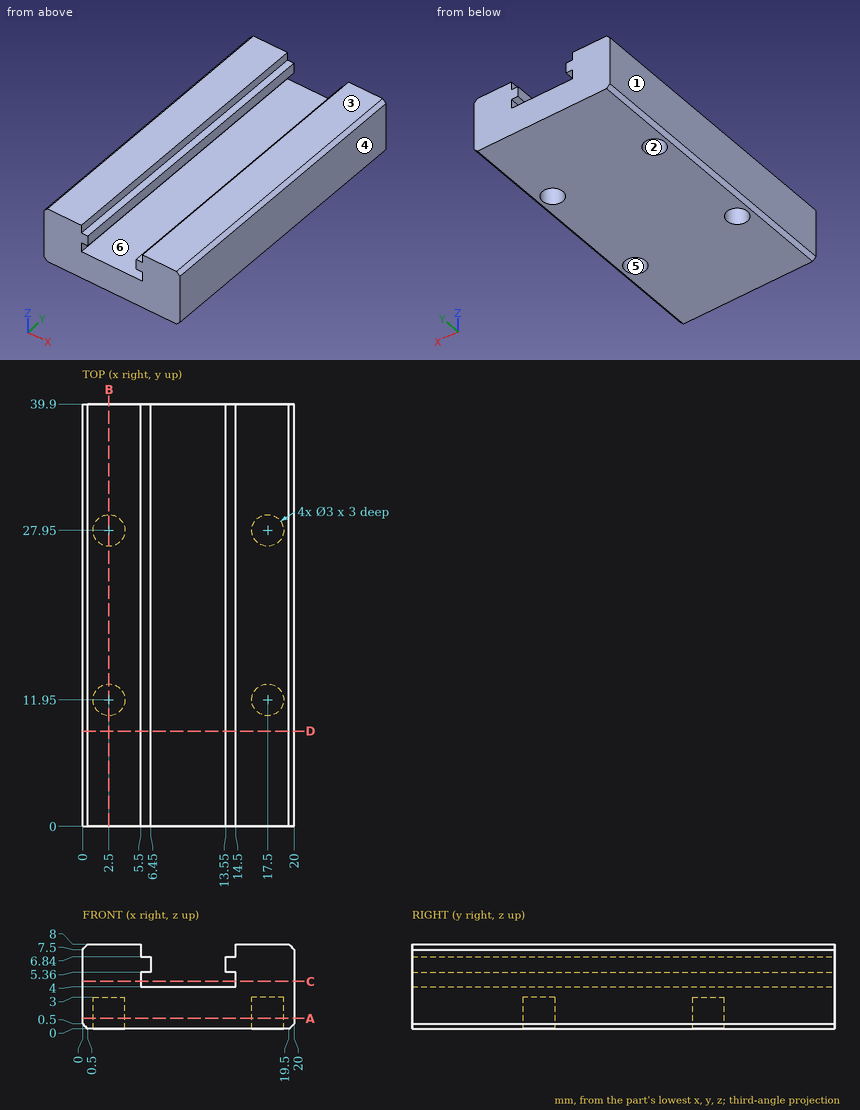
The drawing under review shows one solid part. Ordinate dimensions are in mm from its lowest x, y, z. A direction names the side the tool comes from. Round coordinates to 2 decimals unless told otherwise and drop trailing zeros. Write each loop counter-clockwise with the first axis right and the second up, starting at its lowest first coordinate (ties: lowest second). Pieces come first, ordered by that corner, then holes. Notation, with made-up numbers: (-14.5, -5) - (10.5, -5) arc R27 cw to (10.5, 28) - close; hole circle Ø6 at (69.5, 16). An arc over 180 degrees is marked (long way). Write each question's results on one line, items separated by ' | '.
Item 1: For pin 1 (0.8 mm diameter, centred on x = 6, y = 28, fed in from +Z); pin 2 (1.5 mm diameter, centred on x = 2, y = 27.5, fed in from -Z), all flat-tipped, find the tip position at first contact; note any pin that passes through.
Calculated:
pin 1: stops at z = 6.84 | pin 2: stops at z = 3
Item 2: Take a section at A-A on z = 1. State the section outline as (x, y) points, then the cut area to 3 significant figures.
Calculated:
outline: (0, 0) - (20, 0) - (20, 39.9) - (0, 39.9) - close; hole circle Ø3 at (2.5, 11.95); hole circle Ø3 at (2.5, 27.95); hole circle Ø3 at (17.5, 11.95); hole circle Ø3 at (17.5, 27.95) | area: 770 mm^2
Item 3: Take a section at C-C on z = 4.5. State the section outline as (x, y) points, then the cut area to 3 significant figures.
Calculated:
outline: (0, 0) - (5.5, 0) - (5.5, 39.9) - (0, 39.9) - close; (14.5, 0) - (20, 0) - (20, 39.9) - (14.5, 39.9) - close | area: 439 mm^2
Item 4: Draft analysis for pull direction X (two halves, no side actions). For the marked faces 1, 2 and 3, state which applies: pulls with the +X half, pulls with the -X half, needs draft (parallel to the pull), parting line crosses it, or undercut.
Calculated:
face 1: pulls with the -X half | face 2: undercut | face 3: needs draft
Item 5: Take a section at B-B on x = 2.5. State the section outline as (y, z) points, then the cut area to 3 significant figures.
Calculated:
outline: (0, 0) - (10.45, 0) - (10.45, 3) - (13.45, 3) - (13.45, 0) - (26.45, 0) - (26.45, 3) - (29.45, 3) - (29.45, 0) - (39.9, 0) - (39.9, 8) - (0, 8) - close | area: 301 mm^2
Item 6: For the marked faces 4, 5 and 6, list the 3-axis set-ups (+Z, -Z, +X, -X, +Y, -Y) from which the entire face can be reached by the end or side of a thin tool; tool diameter is ignored.
Calculated:
face 4: +Z, -Z, +X, +Y, -Y | face 5: -Z | face 6: +Y, -Y
Item 7: To check wall thickness, follow line 1 along Y through (x, z) = (2.5, 0.8); line 2 along X through (y, z) = (16.5, 6.75); line 3 along X through (y, z) = (27, 4.5). State the ranges of each line that lie inside material, in increasing order. Write a range as from..to.
Calculated:
line 1: y = 0..10.45, 13.45..26.45, 29.45..39.9 | line 2: x = 0..6.45, 13.55..20 | line 3: x = 0..5.5, 14.5..20
Item 8: Take a section at D-D on y = 9. State the section outline as (x, z) points, then the cut area to 3 significant figures.
Calculated:
outline: (0, 0.5) - (0.5, 0) - (19.5, 0) - (20, 0.5) - (20, 7.5) - (19.5, 8) - (14.5, 8) - (14.5, 6.84) - (13.55, 6.84) - (13.55, 5.36) - (14.5, 5.36) - (14.5, 4) - (5.5, 4) - (5.5, 5.36) - (6.45, 5.36) - (6.45, 6.84) - (5.5, 6.84) - (5.5, 8) - (0.5, 8) - (0, 7.5) - close | area: 126 mm^2
